Autodesk Inventor part; units mm, degrees
ref_plane "YZ Plane" through (0, 0, 0) normal (1, 0, 0) x (0, 1, 0)
ref_plane "XZ Plane" through (0, 0, 0) normal (0, 1, 0) x (-1, 0, 0)
ref_plane "XY Plane" through (0, 0, 0) normal (0, 0, 1) x (1, 0, 0)
sketch "Sketch1" plane through (0, 0, 0) normal (0, 1, 0) x (-1, 0, 0)
  circle A0 centre (0, 0) radius 35.17
  circle A1 centre (0, 0) radius 14.25
  line L0 (14.25, 0) -> (35.17, 0)
  line L1 (-17.4726, 17.4726) -> (36, -36)
  line L2 (0, 0) -> (50.9117, 0) construction
  line L3 (0, 0) -> (0, -35.17)
  line L4 (0, -35.17) -> (0, -14.25)
  circle A2 centre (0, 0) radius 24.71
  circle A3 centre (17.4726, -17.4726) radius 6
  line L5 (17.4726, 17.4726) -> (-36, -36)
  circle A4 centre (-17.4726, -17.4726) radius 6
  circle A5 centre (17.4726, 17.4726) radius 6
  circle A6 centre (-17.4726, 17.4726) radius 6
  point P0 (0, -24.71)
  dimension "d0" = 70.34
  dimension "d1" = 28.5
  dimension "d2" = 45
  dimension "d20" = 12
  dimension "d21" = 12
  dimension "d22" = 12
  dimension "d23" = 12
extrude "Extrusion1" add sketch "Sketch1" along normal blind 2.5 contours L0 A2 A5 A6 A4 L5 A0 | A0 L1 A3 A2 L0 | L5 A4 A2 L3 A0 | A0 L3 A2 A3 L1 | A2 A3 L1 A1 L0 | L0 A1 L5 A5 A2 | A2 A4 L5 A1 L3 | L3 A1 L1 A3 A2 | A2 A6 L1 A1 L5 A4 | A1 L1 A6 A2 A5 L5
sketch "Sketch2" plane through (0, 2.5, 0) normal (0, 1, 0) x (1, 0, 0)
  circle A0 centre (0, 0) radius 35.17
  circle A1 centre (0, 0) radius 14.25
  line L0 (-14.25, 0) -> (-35.17, 0)
  line L1 (-24.71, 0) -> (-24.71, 1.25)
  line L2 (-24.71, 1.25) -> (-24.71, -1.25)
  line L3 (-24.71, 1.25) -> (-31.71, 1.25)
  line L4 (-24.71, 1.25) -> (-17.71, 1.25)
  line L5 (-17.71, 1.25) -> (-17.71, -1.25)
  line L6 (-17.71, -1.25) -> (-31.71, -1.25)
  line L7 (-31.71, -1.25) -> (-31.71, 1.25)
  line L8 (-1.25, -24.71) -> (-1.25, -17.71)
  line L9 (-1.25, -17.71) -> (1.25, -17.71)
  line L10 (1.25, -17.71) -> (1.25, -31.71)
  line L11 (1.25, -31.71) -> (-1.25, -31.71)
  line L12 (-1.25, -24.71) -> (-1.25, -31.71)
  line L13 (24.71, -1.25) -> (17.71, -1.25)
  line L14 (17.71, -1.25) -> (17.71, 1.25)
  line L15 (17.71, 1.25) -> (31.71, 1.25)
  line L16 (31.71, 1.25) -> (31.71, -1.25)
  line L17 (24.71, -1.25) -> (31.71, -1.25)
  line L18 (1.25, 24.71) -> (1.25, 17.71)
  line L19 (1.25, 17.71) -> (-1.25, 17.71)
  line L20 (-1.25, 17.71) -> (-1.25, 31.71)
  line L21 (-1.25, 31.71) -> (1.25, 31.71)
  line L22 (1.25, 24.71) -> (1.25, 31.71)
  dimension "d24" = 1.25
  dimension "d25" = 2.5
  dimension "d26" = 7
  dimension "d27" = 7
  dimension "d30" = 360
extrude "Extrusion2" cut sketch "Sketch2" against normal blind 22.25 contours L7 L3 L1 L0 | L0 L2 L6 L7 | L1 L4 L5 L0 | L0 L5 L6 L2 | L8 L9 L10 L11 L12 | L13 L14 L15 L16 L17 | L18 L19 L20 L21 L22
pattern_circular "Circular Pattern1" count 4 over 360 about axis through (0, -10, 0) along (0, 1, 0) of "Extrusion2"
properties part number "Anillo de Centrado" material "MDF Medium Density Fiberboard"
Read the model definition and answer for the solid it produces. Units are mm, in the model's axes. Give positions to 0.01 mm unless a question says otherwise; leave off trailing zeros. Loops run counter-clockwise (first coordinate to the right, second up) from the corner with the lowest first, then second, coordinate; pieces in that order, holes last. Notation, with made-up numbers: (69.25, 55.5) -> (124.25, 55.5) arc R20 cw to (124.25, 80.5) -> close; hole circle Ø4 at (73, 2). An arc over 180 degrees is marked (long way). Use a Markdown table: item, result.
Q1. Section C-C, the plane y = 2.1 is taken. Count the separate pieces of the cut face and the enclosed holes in it, then the cut area to 3 significant figures.
Solved:
| item | result |
|---|---|
| separate pieces | 1 |
| enclosed holes | 9 |
| area | 2,660 mm^2 |
Q2. Section A-A, the plane z = 0 is taken. Determine the outline of the cut face in (x, y), then the cut area to 3 significant figures.
Solved:
| item | result |
|---|---|
| outline | (-35.17, 0) -> (-31.71, 0) -> (-31.71, 2.5) -> (-35.17, 2.5) -> close; (-17.71, 0) -> (-14.25, 0) -> (-14.25, 2.5) -> (-17.71, 2.5) -> close; (14.25, 0) -> (17.71, 0) -> (17.71, 2.5) -> (14.25, 2.5) -> close; (31.71, 0) -> (35.17, 0) -> (35.17, 2.5) -> (31.71, 2.5) -> close |
| area | 34.6 mm^2 |
Q3. Each of these flat-tipped pins is pushed along its axis until it touches: pin 1 (1.2 mm diameter, centred on x = -26.5, y = 0.5, fed in from +Z); pin 2 (0.8 mm diameter, centred on x = -0.5, y = 1.5, fed in from -Z); pin 3 (1 mm diameter, centred on y = 0.5, z = 4.5, fed in from -X); pin 4 (9.5 mm diameter, centred on x = -17.47, z = -17.47, fed in from -Y). Where does it stop, or does it pass through?
Solved:
| item | result |
|---|---|
| pin 1 | stops at z = 23.79 |
| pin 2 | stops at z = -35.17 |
| pin 3 | stops at x = -34.94 |
| pin 4 | passes through |
Q4. Determine the mould class of faces 1 (the face through (16, 2.5, 0)), 2 (the face through (7.624, 1.232, 34.334)), 3 (the face through (0, 1, 31.71)) for opening direction X: pulls with the +X half, pulls with the -X half, needs draft (parallel to the pull), parting line crosses it, or undercut.
Solved:
| item | result |
|---|---|
| face 1 | needs draft |
| face 2 | parting line crosses it |
| face 3 | undercut |
Q5. Find the intervals of material crossed by line 1 along Z through (x, y) = (0, 0.6); line 2 along X through (y, z) = (1.1, 21), in increasing order.
Solved:
| item | result |
|---|---|
| line 1 | z = -35.17 to -31.71, -17.71 to -14.25, 14.25 to 17.71, 31.71 to 35.17 |
| line 2 | x = -28.21 to -22.33, -12.62 to -1.25, 1.25 to 12.62, 22.33 to 28.21 |
Q6. Section D-D, the plane z = -15.5 is taken. Determine the outline of the cut face in (x, y).
Solved:
| item | result |
|---|---|
| outline | (-31.57, 0) -> (-23.14, 0) -> (-23.14, 2.5) -> (-31.57, 2.5) -> close; (-11.81, 0) -> (11.81, 0) -> (11.81, 2.5) -> (-11.81, 2.5) -> close; (23.14, 0) -> (31.57, 0) -> (31.57, 2.5) -> (23.14, 2.5) -> close |
Q7. Section B-B, the plane x = 0 is taken. Determine the outline of the cut face in (y, z), then the cut area to 3 significant figures.
Solved:
| item | result |
|---|---|
| outline | (0, -35.17) -> (2.5, -35.17) -> (2.5, -31.71) -> (0, -31.71) -> close; (0, -17.71) -> (2.5, -17.71) -> (2.5, -14.25) -> (0, -14.25) -> close; (0, 14.25) -> (2.5, 14.25) -> (2.5, 17.71) -> (0, 17.71) -> close; (0, 31.71) -> (2.5, 31.71) -> (2.5, 35.17) -> (0, 35.17) -> close |
| area | 34.6 mm^2 |
